from build123d import *

# Parameters (mm, degrees)
F1_DEPTH = 25.4
F2_SIZE  = 10.16


with BuildPart() as f1:
    # F0 (on Front) → F1 (new body)
    with BuildSketch(Plane.XZ):
        Polygon((14.401741, 19.822295), (0, 64.146296), (-14.401741, 19.822295), (-61.006753, 19.822295), (-23.302506, -7.571443), (-37.704247, -51.895443), (0, -24.501705), (37.704247, -51.895443), (23.302506, -7.571443), (61.006753, 19.822295), align=None)
    extrude(amount=F1_DEPTH)

    # F2
    f2_edges = [f1.edges().sort_by_distance(p)[0] for p in [
        (42.154629, -25.4, 6.125426),
        (37.704247, -25.4, 19.822295),
        (7.20087, -25.4, 41.984296),
        (-7.20087, -25.4, 41.984296),
        (-37.704247, -25.4, 19.822295),
        (-42.154629, -25.4, 6.125426),
        (-30.503376, -25.4, -29.733443),
        (-18.852123, -25.4, -38.198574),
        (18.852123, -25.4, -38.198574),
        (30.503376, -25.4, -29.733443),
        (42.154629, 0, 6.125426),
        (37.704247, 0, 19.822295),
        (7.20087, 0, 41.984296),
        (-7.20087, 0, 41.984296),
        (-37.704247, 0, 19.822295),
        (-42.154629, 0, 6.125426),
        (-30.503376, 0, -29.733443),
        (-18.852123, 0, -38.198574),
        (18.852123, 0, -38.198574),
        (30.503376, 0, -29.733443),
    ]]
    chamfer(f2_edges, length=F2_SIZE)


solid = f1.part
Work out the finished part from the listing and answer in its coordinate system (mm). A direction names the side the tool comes from. Round coordinates to 2 decimals unless told otherwise and drop trailing zeros. Order: outer loops, then holes, each group sorted by start corner. A loop starts at its lowest first (then second) coordinate and runs counter-clockwise, first axis right, second up. Notation, with made-up numbers: M 10,45 L 42,45 A21 ccw 42,73 Z; hole C 14,-6.75 d1. An arc over 180 degrees is marked long. Put each result on its own line as item: value. Start each with the question number.
Q1. Flat-ended cylindrical pins translate along their axes: pin 1 (1 mm diameter, centred on y = -18.5, z = -30.5, fed in from +X); pin 2 (1 mm diameter, centred on x = 29.5, z = 13, fed in from +Y); pin 3 (5.5 mm diameter, centred on x = -28.5, y = -13, fed in from +Z). Find the tip coordinate at first contact, or state that the pin passes through.
Q2. For a pull along X with two mould halves and no side action, classify faces 6 (the flat face through (-31.594, -20.391, 4.82)), 7 (the flat face through (22.73, -5.01, -22.47)), 8 (the flat face through (28.39, -20.39, 14.67)), 9 (the flat face through (-19.116, -12.664, -38.39)) as pulls with the +X half, pulls with the -X half, needs draft (parallel to the pull), parting line crosses it, or undercut.
Q3. Section B-B, the plane y = -13 is taken. Write down the section's boundary in (x, z).
Q4. A tool of negligible diameter and unlimited length cuts with its end or side. For faces 1 (the flat face through (-23.57, -19.26, -21.4)), 2 (the flat face through (-23.57, -6.14, -21.4)), 3 (the flat face through (30.604, -12.664, -30.044)), 4 (the flat face through (13.1, -19.3, -29)), 5 (the flat face through (-37, -13, 19.822)), from which of +Z, -Z, +X, -X, +Y, -Y can it reach the whole face along a straight path? Write none if from no direction.
Q5. Section D-D, the plane x = 51.5 is taken. Write down the section's boundary in (y, z).
Q6. Section C-C, the plane z = -9 is taken. Write down the section's boundary in (x, y).
Q7. Straight lines are drawn through the part: L1, parallel to X at y = -17.25, z = -35.5; L2, parallel to X at y = -5.5, z = -20; L3, parallel to X at y = -11.75, z = 52. For each, find the intervals that lie inside material, in ascending order. Write a range as [from, to].
Q8. Section A-A, the plane x = 31.5 is taken. Write down the section's boundary in (y, z).
Findings below:
1. pin 1: stops at x = 27.87
1. pin 2: stops at y = -2.84
1. pin 3: stops at z = 19.82
2. face 6: pulls with the -X half
2. face 7: pulls with the +X half
2. face 8: needs draft
2. face 9: undercut
3. outline: M -61.01,19.82 L -23.3,-7.57 L -37.7,-51.9 L 0,-24.5 L 37.7,-51.9 L 23.3,-7.57 L 61.01,19.82 L 14.4,19.82 L 0,64.15 L -14.4,19.82 Z
4. face 1: -X, -Y
4. face 2: -X, +Y
4. face 3: +X, +Y, -Y
4. face 4: -Z, -Y
4. face 5: +Z, -X, +Y, -Y
5. outline: M -18.33,16.73 L -15.24,12.92 L -10.16,12.92 L -7.07,16.73 L -10.16,19.82 L -15.24,19.82 Z
6. outline: M -23.77,-15.24 L -13.08,-25.4 L 13.08,-25.4 L 23.77,-15.24 L 23.77,-10.16 L 13.08,0 L -13.08,0 L -23.77,-10.16 Z
7. L1: x = [-30.26, -18.56], [18.56, 30.26]
7. L2: x = [-22.44, -1.73], [1.73, 22.44]
7. L3: x = [-3.95, 3.95]
8. outline: M -24.83,10.23 L -15.24,-1.62 L -10.16,-1.62 L -0.57,10.23 L -10.16,19.82 L -15.24,19.82 Z; M -18.5,-43.36 L -15.24,-47.39 L -10.16,-47.39 L -6.9,-43.36 L -10.16,-32.8 L -15.24,-32.8 Z
